from build123d import *

# Parameters (mm, degrees)
F0_W     = 69.85
F0_H     = 12.7
F1_DEPTH = 25.4
F2_R     = 12.7
F2_R_2   = 6.35
F3_DEPTH = 25.4
F4_DEPTH = 25.4
F6_DEPTH = 25.4


with BuildPart() as f1:
    # F0 (on Front) → F1 (new body)
    with BuildSketch(Plane.XZ):
        with Locations((34.925, 6.35)):
            Rectangle(F0_W, F0_H)
    extrude(amount=F1_DEPTH)

    # F2 (on face) → F3 (join)
    with BuildSketch(Plane.XY.offset(12.7)):
        with Locations((12.7, -12.7)):
            Circle(F2_R)
        with Locations((12.7, -12.7)):
            Circle(F2_R_2, mode=Mode.SUBTRACT)
    extrude(amount=F3_DEPTH)

    # F4 (cut): faces of the model
    f4_faces = [f1.faces().sort_by_distance(p)[0] for p in [
        (2.8367728246, -22.5632271754, 12.7),
        (2.8367728246, -2.8367728246, 12.7),
    ]]
    extrude(f4_faces, amount=-F4_DEPTH, mode=Mode.SUBTRACT)

    # F5 (on face) → F6 (cut)
    with BuildSketch(Plane.XY.offset(12.7)):
        with BuildLine():
            ThreePointArc((38.1, -19.05), (42.5901280605, -17.1901280605), (44.45, -12.7))
            ThreePointArc((44.45, -12.7), (42.5901280605, -8.2098719395), (38.1, -6.35))
            ThreePointArc((38.1, -6.35), (31.75, -12.7), (38.1, -19.05))
        make_face()
        with BuildLine():
            ThreePointArc((38.1, -6.35), (42.5901280605, -8.2098719395), (44.45, -12.7))
            ThreePointArc((44.45, -12.7), (42.5901280605, -17.1901280605), (38.1, -19.05))
            Line((38.1, -19.05), (57.15, -19.05))
            ThreePointArc((57.15, -19.05), (50.8, -12.7), (57.15, -6.35))
            Line((57.15, -6.35), (38.1, -6.35))
        make_face()
        with BuildLine():
            ThreePointArc((63.5, -12.7), (61.6401280605, -8.2098719395), (57.15, -6.35))
            ThreePointArc((57.15, -6.35), (50.8, -12.7), (57.15, -19.05))
            ThreePointArc((57.15, -19.05), (61.6401280605, -17.1901280605), (63.5, -12.7))
        make_face()
        with BuildLine():
            ThreePointArc((57.15, 0), (66.1302561211, -3.7197438789), (69.85, -12.7))
            Line((69.85, -12.7), (69.85, 0))
            Line((69.85, 0), (57.15, 0))
        make_face()
        with BuildLine():
            ThreePointArc((69.85, -12.7), (66.1302561211, -21.6802561211), (57.15, -25.4))
            Line((57.15, -25.4), (69.85, -25.4))
            Line((69.85, -25.4), (69.85, -12.7))
        make_face()
    extrude(amount=-F6_DEPTH, mode=Mode.SUBTRACT)


solid = f1.part
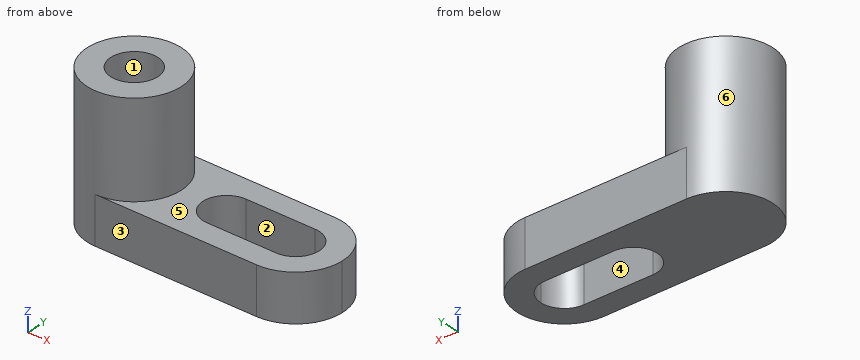
Work out the finished part from the listing and answer in its coordinate system (mm). Face numbers are marked on the shaded views. A direction names the side the tool comes from. Coordinates: 2 decimals unless noted, no trailing zeros. Loops run counter-clockwise (first coordinate to the right, second up) from the corner with the lowest first, then second, coordinate; pieces in that order, holes last. Notation, with made-up numbers: (-24.75, 26.25) -> (-17.75, 26.25) arc R27 cw to (-17.75, 47.25) -> close; hole circle Ø2 at (-5, 0.25). An arc over 180 degrees is marked (long way). Write each question's results on one line, items separated by ' | '. Start each with the question number.
1) Find section D-D on z = 20. Determine the outline of the cut face in (x, y).
2) Consider line 1 along Y through (x, z) = (12.7, 26.75); line 2 along Z through (x, y) = (44.5, -24); line 3 along X through (y, z) = (-15.25, 25). Determine where each line is inside the solid, lowest interval first.
3) Find section C-C on x = 17. Determine the outline of the cut face in (y, z).
4) The mould has two halves that part along X. Classify the marked faces 4, 5 and 6: pulls with the +X half, pulls with the -X half, needs draft (parallel to the pull), parting line crosses it, or undercut.
5) Find section A-A on y = -10. Determine the outline of the cut face in (x, z), then the cut area to 3 significant figures.
6) Find section B-B on x = 59. Determine the outline of the cut face in (y, z), then the cut area to 3 significant figures.
7) For the marked faces 1, 2 and 3, determine the directions among +Z, -Z, +X, -X, +Y, -Y from which every point of the face is accessible in a straight line to the end or side of a thin tool.
8) Flat-ended cylindrical pins translate along their axes: P1, Ø10, axis at y = -6, z = 14, coming from the +X side; P2, Ø2, axis at y = -22, z = 29.5, coming from the +X side; P3, Ø4, axis at y = -19.5, z = 27.5, coming from the +X side. Find the tip coordinate at first contact, or state that the pin passes through.
Response values:
1) outline: circle Ø25.4 at (12.7, -12.7); hole circle Ø12.7 at (12.7, -12.7)
2) line 1: y = -25.4 to -19.05, -6.35 to 0 | line 2: z = 0 to 12.7 | line 3: x = 0.26 to 6.88, 18.52 to 25.14
3) outline: (-25.4, 0) -> (0, 0) -> (0, 12.7) -> (-0.75, 12.7) -> (-0.75, 38.1) -> (-8.03, 38.1) -> (-8.03, 12.7) -> (-17.37, 12.7) -> (-17.37, 38.1) -> (-24.65, 38.1) -> (-24.65, 12.7) -> (-25.4, 12.7) -> close
4) face 4: undercut | face 5: needs draft | face 6: parting line crosses it
5) outline: (0.29, 0) -> (32.35, 0) -> (32.35, 12.7) -> (25.11, 12.7) -> (25.11, 38.1) -> (18.45, 38.1) -> (18.45, 12.7) -> (6.95, 12.7) -> (6.95, 38.1) -> (0.29, 38.1) -> close; (62.9, 0) -> (69.56, 0) -> (69.56, 12.7) -> (62.9, 12.7) -> close | area: 830 mm^2
6) outline: (-25.26, 0) -> (-18.77, 0) -> (-18.77, 12.7) -> (-25.26, 12.7) -> close; (-6.63, 0) -> (-0.14, 0) -> (-0.14, 12.7) -> (-6.63, 12.7) -> close | area: 165 mm^2
7) face 1: +Z | face 2: +Z, -Z | face 3: +Z, -Z, +X, -X, -Y
8) P1: stops at x = 69.71 | P2: stops at x = 22.31 | P3: stops at x = 24.46
